```python
from build123d import *

# Parameters (mm, degrees)
SWEEP2_PROFILE_R   = 7.5
SKETCH41_W         = 5.5
SKETCH41_H         = 14
CUT_EXTRUDE1_DEPTH = 7.5
SKETCH40_R         = 2
CUT_EXTRUDE2_DEPTH = 65
SKETCH42_R         = 2.5
CUT_EXTRUDE3_DEPTH = 10


with BuildPart() as part:
    # Sweep2: sweep along a path in Sketch1
    with BuildLine(Plane.XY) as sweep2_path:
        Line((-60, 350), (-60, 10))
        ThreePointArc((-60, 10), (-57.071067812, 2.928932188), (-50, 0))
        Line((-50, 0), (50, 0))
        ThreePointArc((50, 0), (57.071067812, 2.928932188), (60, 10))
        Line((60, 10), (60, 350))
    # Sweep2 profile (on start of the path) → Sweep2 (sweep)
    with BuildSketch(Plane(origin=(-60, 350, 0), x_dir=(-1, 0, 0), z_dir=(0, -1, 0))):
        Circle(SWEEP2_PROFILE_R)
    sweep(path=sweep2_path.line)

    # Sketch41 → Cut-Extrude1 (cut, symmetric)
    with BuildSketch(Plane.XY):
        with Locations((-64.75, 343)):
            Rectangle(SKETCH41_W, SKETCH41_H)
        with Locations((-55.25, 343)):
            Rectangle(SKETCH41_W, SKETCH41_H)
        with Locations((55.25, 343)):
            Rectangle(SKETCH41_W, SKETCH41_H)
        with Locations((64.75, 343)):
            Rectangle(SKETCH41_W, SKETCH41_H)
    extrude(amount=CUT_EXTRUDE1_DEPTH, both=True, mode=Mode.SUBTRACT)

    # Sketch40 → Cut-Extrude2 (cut, symmetric)
    with BuildSketch(Plane(origin=(0, 0, 0), x_dir=(0, 0, -1), z_dir=(1, 0, 0))):
        with Locations((0, 342)):
            Circle(SKETCH40_R)
    extrude(amount=CUT_EXTRUDE2_DEPTH, both=True, mode=Mode.SUBTRACT)

    # Sketch42 → Cut-Extrude3 (cut, symmetric)
    with BuildSketch(Plane.XY):
        Circle(SKETCH42_R)
    extrude(amount=CUT_EXTRUDE3_DEPTH, both=True, mode=Mode.SUBTRACT)


solid = part.part
```
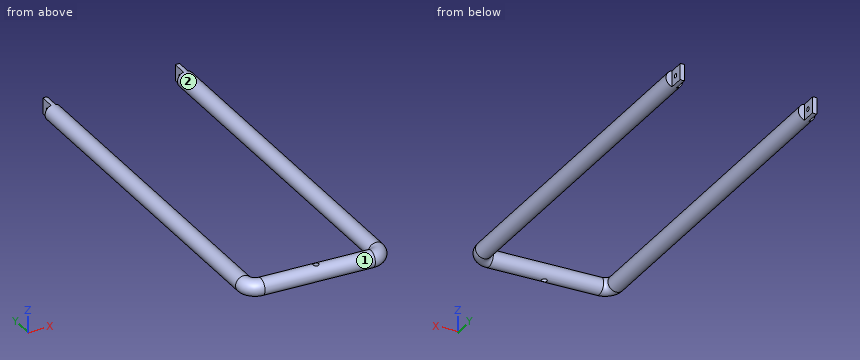
CAD build for the part. Positions are in the model's coordinates, mm. Face numbers are marked on the shaded views. Round coordinates to 2 decimals unless told otherwise and drop trailing zeros. Order: outer loops, then holes, each group sorted by start corner. A loop starts at its lowest first (then second) coordinate and runs counter-clockwise, first axis right, second up. Notation, with made-up numbers: (-13, 24.25) - (32, 24.25) arc R22 cw to (32, 62.25) - close; hole circle Ø8 at (27.5, -33.5). An arc over 180 degrees is marked (long way). Use CSV: the item, a comma, the result in double quotes. Start each with the question number.
1) Saw through at A-A (y = 78.5). List the corners of the cut face in (x, z).
2) Saw through at B-B (x = 22). List the corners of the cut face in (y, z), and give its area (3 significant figures).
3) Pin check, flat tips, straight feed: pin 1 Ø4 at (x, y) = (-52, 287) entering from -Z; pin 2 Ø6.5 at (y, z) = (342, 0) entering from -X; pin 3 Ø7 at (y, z) = (343.5, 1) entering from +X; pin 4 Ø8 at (y, z) = (269, -1.5) entering from -X. Stop position of each tip, or through.
4) Wall check: L1, parallel to X at y = 89, z = 1; L2, parallel to Y at x = 0, z = 0; L3, parallel to Z at x = 60, y = 342. Give the ranges that are in metal, low to high. Write a range as [from, to].
5) Two-plate mould, pull along X, no slides. Class the marked faces 1 and 2: pulls with the +X half, pulls with the -X half, needs draft (parallel to the pull), parting line crosses it, or undercut.
Values follow:
1,outline,"circle Ø15 at (-60, 0); circle Ø15 at (60, 0)"
2,outline,"circle Ø15 at (0, 0)"
2,area,"177 mm2"
3,pin 1,"stops at z = -4.5"
3,pin 2,"stops at x = -62"
3,pin 3,"stops at x = 62"
3,pin 4,"stops at x = -67.5"
4,L1,"x = [-67.43, -52.57], [52.57, 67.43]"
4,L2,"y = [-7.5, -2.5], [2.5, 7.5]"
4,L3,"z = [-7.5, -2], [2, 7.5]"
5,face 1,"undercut"
5,face 2,"undercut"
